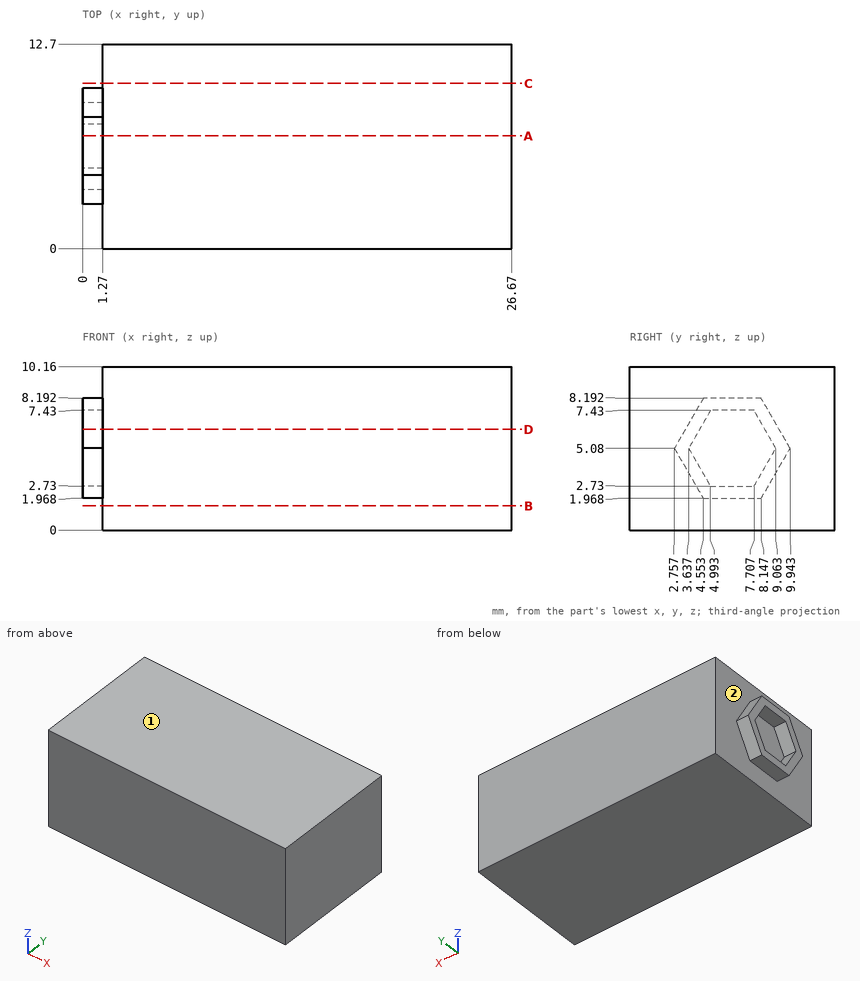
The drawing under review shows one solid part. Ordinate dimensions are in mm from its lowest x, y, z. A direction names the side the tool comes from. Give positions to 0.01 mm unless a question says otherwise; leave off trailing zeros. Order: outer loops, then holes, each group sorted by start corner. A loop starts at its lowest first (then second) coordinate and runs counter-clockwise, first axis right, second up. Notation, with made-up numbers: (25.25, -28.75) - (81.25, -28.75) arc R21 ccw to (81.25, -0.75) - close; hole circle Ø2 at (30.25, 43). An arc over 180 degrees is marked (long way). Answer as a JSON object with one key per item and string values. Group by question number.
Item 1: Take a section at B-B on z = 1.5. Give the boundary of the cut face in (x, y), and give its area (3 significant figures).
Item 2: Take a section at C-C on y = 10.25. Give the boundary of the cut face in (x, z), and give its area (3 significant figures).
Item 3: Clearance check with flat-ended pins moving along their axes: pin 1 Ø3 at (y, z) = (7.5, 2) entering from -X; pin 2 Ø4 at (y, z) = (10.5, 1.5) entering from -X. State where each tip first meets the part, or that it passes through.
Item 4: Machinability: for the marked faces 1 and 2, which of the approach directions +Z, -Z, +X, -X, +Y, -Y give a long, thin tool a straight path to every point of the face, cutting with its end or side? Answer none if there is none.
Item 5: Take a section at A-A on y = 7. Give the boundary of the cut face in (x, z), and give its area (3 significant figures).
Item 6: Wall thickness on line 1 along X through (y, z) = (2, 9.75): over which ranges is the line inside the solid? List them lowest first.
Item 7: Take a section at D-D on z = 6.25. Give the boundary of the cut face in (x, y).
Reported:
{
 "1": {"outline": "(1.27, 0) - (26.67, 0) - (26.67, 12.7) - (1.27, 12.7) - close", "area": "323 mm^2"},
 "2": {"outline": "(1.27, 0) - (26.67, 0) - (26.67, 10.16) - (1.27, 10.16) - close", "area": "258 mm^2"},
 "3": {"pin 1": "x = 0", "pin 2": "x = 1.27"},
 "4": {"face 1": "+Z, +X, -X, +Y, -Y", "face 2": "-X"},
 "5": {"outline": "(0, 1.97) - (1.27, 1.97) - (1.27, 0) - (26.67, 0) - (26.67, 10.16) - (1.27, 10.16) - (1.27, 8.19) - (0, 8.19) - (0, 7.43) - (1.27, 7.43) - (1.27, 2.73) - (0, 2.73) - close", "area": "260 mm^2"},
 "6": {"line 1": "1.27 to 26.67"},
 "7": {"outline": "(0, 3.43) - (1.27, 3.43) - (1.27, 0) - (26.67, 0) - (26.67, 12.7) - (1.27, 12.7) - (1.27, 9.27) - (0, 9.27) - (0, 8.39) - (1.27, 8.39) - (1.27, 4.31) - (0, 4.31) - close"}
}
